from build123d import *

# Parameters (mm, degrees)
REVOLU_O1_ANGLE            = 180
ESBO_O6_R                  = 20
CORTE_EXTRUS_O3_DEPTH      = 130.903810568
ESBO_O7_R                  = 7.5
CORTE_EXTRUS_O4_DEPTH      = 129.354976586
CORTE_EXTRUS_O5_DEPTH      = 50
CORTE_EXTRUS_O5_DEPTH_BACK = 44
ESBO_O8_W                  = 70
ESBO_O8_H                  = 12.551087697
ESBO_O9_R                  = 1
CORTE_EXTRUS_O6_DEPTH      = 126.312510747
SKETCH2_R                  = 8.2
CUT_EXTRUDE3_DEPTH         = 30
SKETCH4_R                  = 1
CUT_EXTRUDE4_DEPTH         = 20


with BuildPart() as part:
    # Esbo_o1 → Revolu_o1 (revolve)
    with BuildSketch(Plane.XY):
        with BuildLine():
            Line((-60, 0), (-75, 0))
            ThreePointArc((-75, 0), (0, 75), (75, 0))
            Line((75, 0), (60, 0))
            ThreePointArc((60, 0), (0, 60), (-60, 0))
        make_face()
    revolve(axis=Axis((-60, 0, 0), (-1, 0, 0)), revolution_arc=REVOLU_O1_ANGLE)

    # Esbo_o6 → Corte-extrus_o3 (cut, through all)
    with BuildSketch(Plane.XY):
        Circle(ESBO_O6_R)
    extrude(amount=-CORTE_EXTRUS_O3_DEPTH, mode=Mode.SUBTRACT)

    # Esbo_o7 → Corte-extrus_o4 (cut, through all)
    with BuildSketch(Plane(origin=(0, 0, 0), x_dir=(0, 0, -1), z_dir=(1, 0, 0))):
        Circle(ESBO_O7_R)
    extrude(amount=-CORTE_EXTRUS_O4_DEPTH, mode=Mode.SUBTRACT)

    # Esbo_o8 → Corte-extrus_o5 (cut, two sides: drawn at the far end of the back side and taken through both)
    with BuildSketch(Plane(origin=(0, 0, 0), x_dir=(1, 0, 0), z_dir=(0, 1, 0)).offset(-CORTE_EXTRUS_O5_DEPTH_BACK)):
        with Locations((0, 73.008034748)):
            Rectangle(ESBO_O8_W, ESBO_O8_H)
    extrude(amount=CORTE_EXTRUS_O5_DEPTH + CORTE_EXTRUS_O5_DEPTH_BACK, mode=Mode.SUBTRACT)

    # Esbo_o9 → Corte-extrus_o6 (cut, through all)
    with BuildSketch(Plane(origin=(0, 0, -66.7324909), x_dir=(-1, 0, 0), z_dir=(0, 0, -1))):
        with Locations((-26, 0)):
            Circle(ESBO_O9_R)
        with Locations((0, 26)):
            Circle(ESBO_O9_R)
        with Locations((26, 0)):
            Circle(ESBO_O9_R)
        with Locations((0, -26)):
            Circle(ESBO_O9_R)
    extrude(amount=-CORTE_EXTRUS_O6_DEPTH, mode=Mode.SUBTRACT)

    # Sketch2 → Cut-Extrude3 (cut)
    with BuildSketch(Plane(origin=(-74.624057783, 0, 0), x_dir=(0, 0, -1), z_dir=(1, 0, 0))):
        with Locations(Location((25, -9.296175558, 0), (0, 0, 280.330861945))):
            Circle(SKETCH2_R)
        with Locations(Location((25, 12.7, 0), (0, 0, 307.012442237))):
            Circle(SKETCH2_R)
    extrude(amount=CUT_EXTRUDE3_DEPTH, mode=Mode.SUBTRACT)

    # Sketch4 → Cut-Extrude4 (cut)
    with BuildSketch(Plane.XY.offset(10)):
        with Locations((66.5, 0)):
            Circle(SKETCH4_R)
        with Locations((0, -66.5)):
            Circle(SKETCH4_R)
        with Locations((-66.5, 0)):
            Circle(SKETCH4_R)
        with Locations((0, 66.5)):
            Circle(SKETCH4_R)
    extrude(amount=-CUT_EXTRUDE4_DEPTH, mode=Mode.SUBTRACT)


solid = part.part
CAD build for the part. Positions are in the model's coordinates, mm. A direction names the side the tool comes from. Round coordinates to 2 decimals unless told otherwise and drop trailing zeros. Loops run counter-clockwise (first coordinate to the right, second up) from the corner with the lowest first, then second, coordinate; pieces in that order, holes last.
(1) Cut at C-C (z = -24). Give the cut face in (x, y).
(2) Drop flat-ended pins along their axis: pin 1 (8 mm diameter, centred on y = 49.5, z = -51, fed in from -X); pin 2 (6 mm diameter, centred on x = -57.5, y = 43.5, fed in from -Z); pin 3 (0.6 mm diameter, centred on x = 0, y = 66, fed in from +Z). Give the stop position or say it passes through.
(3) Cut at B-B (y = 15). Give the cut face in (x, z).
(4) Two-plate mould, pull along X, no slides. Class faces 4 (the flat face through (15, 15, -66.732)), 5 (the cylindrical face through (-4.336, -19.524, -61.579)): +X half, -X half, draft (parallel to the pull), parting line (faces both ways), or undercut.
(5) Cut at A-A (x = -13). Give the cut face in (y, z), plus the area to 3 significant figures.
(6) Cut at D-D (z = -60.5). Give the cut face in (x, y).
(7) Which spindle directions (+Z, -Z, +X, -X, +Y, -Y) get a long thin tool onto all of the face, cutting with end or side? Do faces 1 (the cylindrical face through (-65.29, -0.16, -7.5)), 2 (the cylindrical face through (-60.245, 13.342, -33.175)), 3 (the flat face through (50, 34, 0)). Say none if no direction does.
(8) Wall check: line 1 along X through (y, z) = (0, -64); line 2 along Y through (x, z) = (-64.5, -25); line 3 along X through (y, z) = (0, -59.5). Give the ranges that are in metal, low to high.
Findings below:
1. outline: (-71.05, -1.16) - (-54.98, -1.16) arc R54.99 cw to (-54.8, 4.56) - (-70.91, 4.56) arc R71.06 ccw to start; (-68.88, -17.43) arc R71.06 ccw (long way) to (-67.93, 20.84) - (-50.89, 20.84) arc R54.99 cw (long way) to (-52.15, -17.43) - close
2. pin 1: stops at x = -33.56
2. pin 2: stops at z = -29.16
2. pin 3: stops at z = -10
3. outline: (-73.48, 0) arc R73.48 ccw to (-71.46, -17.13) - (-55.51, -17.13) arc R58.09 cw to (-58.09, 0) - close; (-65.72, -32.87) arc R73.48 ccw to (-30.77, -66.73) - (-13.23, -66.73) - (-13.23, -56.57) arc R58.09 cw to (-47.9, -32.87) - close; (13.23, -66.73) - (30.77, -66.73) arc R73.48 ccw to (73.48, 0) - (58.09, 0) arc R58.09 cw to (13.23, -56.57) - close
4. face 4: draft
4. face 5: undercut
5. outline: (-73.86, 0) arc R73.86 ccw to (-31.67, -66.73) - (-15.2, -66.73) - (-15.2, -56.57) arc R58.57 cw to (-58.57, 0) - close; (15.2, -66.73) - (31.67, -66.73) arc R73.86 ccw to (73.86, 0) - (58.57, 0) arc R58.57 cw to (15.2, -56.57) - close
5. area: 2,610 mm2
6. outline: circle Ø88.65 at (0, 0); hole circle Ø2 at (-26, 0); hole circle Ø40 at (0, 0); hole circle Ø2 at (0, -26); hole circle Ø2 at (0, 26); hole circle Ø2 at (26, 0)
7. face 1: +Z, -X
7. face 2: -X
7. face 3: +Z, +X, -X, +Y, -Y
8. line 1: x = -39.1 to -27, -25 to -20, 20 to 25, 27 to 39.1
8. line 2: y = -28.98 to -17.5, -1.1 to 4.5, 20.9 to 28.98
8. line 3: x = -45.66 to -27, -25 to -20, 20 to 25, 27 to 45.66
